from build123d import *

# Parameters (mm, degrees)
F0_W     = 15.24
F0_H     = 25.4
F1_DEPTH = 5.08
F2_W     = 5.08
F2_H     = 5.08
F2_H_2   = 10.16
F3_DEPTH = 5.08
F4_R     = 5.08


with BuildPart() as f1:
    # F0 (on Front) → F1 (new body)
    with BuildSketch(Plane.XZ):
        Rectangle(F0_W, F0_H)
    extrude(amount=F1_DEPTH)

    # F2 (on face) → F3 (cut)
    with BuildSketch(Plane.XZ.offset(5.08)):
        with Locations((0, 5.08)):
            Rectangle(F2_W, F2_H)
        with Locations((0, -7.62)):
            Rectangle(F2_W, F2_H_2)
    extrude(amount=-F3_DEPTH, mode=Mode.SUBTRACT)

    # F4
    f4_edges = [f1.edges().sort_by_distance(p)[0] for p in [
        (-7.62, -2.54, 12.7),
        (7.62, -2.54, 12.7),
    ]]
    fillet(f4_edges, radius=F4_R)


solid = f1.part
Could you check a few things on this model? Use its own coordinates, in mm. A direction names the side the tool comes from. Round coordinates to 2 decimals unless told otherwise and drop trailing zeros. Order: outer loops, then holes, each group sorted by start corner. A loop starts at its lowest first (then second) coordinate and runs counter-clockwise, first axis right, second up.
Q1. I'm going to push a flat-ended pin straight in: P1, Ø1.5, axis at x = -0.5, y = -2.5, coming from the -Z side. Where does the tip first touch, or does it pass through?
Geometry says:
P1: stops at z = -2.54
Q2. Please list where these lines run through material, in increasing order: probe 1 along Z at (x, y) = (-0.5, -0.5); probe 2 along X at (y, z) = (-1.4, 3.5); probe 3 along Z at (x, y) = (-2.75, -0.8).
Geometry says:
probe 1: z = -2.54 to 2.54, 7.62 to 12.7
probe 2: x = -7.62 to -2.54, 2.54 to 7.62
probe 3: z = -12.7 to 12.7
Q3. Imagine slicing it at C-C, the plane y = -2.9. List the corners of the cut face in (x, z) for me, then the cut area to 3 significant figures.
Geometry says:
outline: (-7.62, -12.7) - (-2.54, -12.7) - (-2.54, -2.54) - (2.54, -2.54) - (2.54, -12.7) - (7.62, -12.7) - (7.62, 7.62) arc R5.08 ccw to (2.54, 12.7) - (-2.54, 12.7) arc R5.08 ccw to (-7.62, 7.62) - close; hole (-2.54, 2.54) - (2.54, 2.54) - (2.54, 7.62) - (-2.54, 7.62) - close
area: 299 mm2
Q4. Imagine slicing it at B-B, the plane x = 0. List the corners of the cut face in (y, z) for me, then the cut area to 3 significant figures.
Geometry says:
outline: (-5.08, -2.54) - (0, -2.54) - (0, 2.54) - (-5.08, 2.54) - close; (-5.08, 7.62) - (0, 7.62) - (0, 12.7) - (-5.08, 12.7) - close
area: 51.6 mm2
Q5. Which directions (+Z, -Z, +X, -X, +Y, -Y) give clear straight access to the entire face, cutting with the end or side of a thin tool? Please do faces 1 (the face through (0, -3, 2.54)), 2 (the face through (-2.54, -3, -8)), 3 (the face through (5, -3, -12.7)).
Geometry says:
face 1: +Y, -Y
face 2: -Z, +Y, -Y
face 3: -Z, +X, -X, +Y, -Y
Q6. Imagine slicing it at A-A, the plane z = -5.5. List the corners of the cut face in (x, y) for me.
Geometry says:
outline: (-7.62, -5.08) - (-2.54, -5.08) - (-2.54, 0) - (-7.62, 0) - close; (2.54, -5.08) - (7.62, -5.08) - (7.62, 0) - (2.54, 0) - close
Q7. Thinking about a two-plate mould opening in X: for faces 4 (the face through (-7.62, -3, -3)), 5 (the face through (7.62, -3, -3)), 6 (the face through (2.54, -3, -8)), 7 (the face through (0, -3, 12.7)), which applies, released by +X, released by -X, zero draft, split by the parting line, or undercut?
Geometry says:
face 4: released by -X
face 5: released by +X
face 6: undercut
face 7: zero draft
Q8. Imagine slicing it at D-D, the plane z = 9. List the corners of the cut face in (x, y) for me, then the cut area to 3 significant figures.
Geometry says:
outline: (-7.43, -5.08) - (7.43, -5.08) - (7.43, 0) - (-7.43, 0) - close
area: 75.5 mm2
